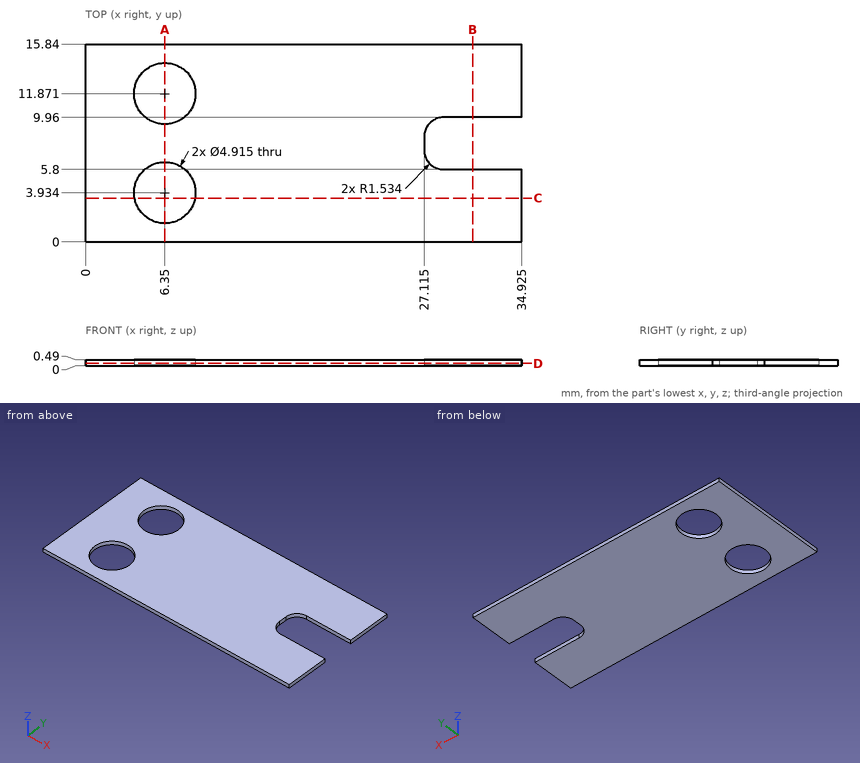
Check sheet for the drawn part. Datum: minimum x, y, z corner. Units: mm. Coordinates: 2 decimals unless noted, no trailing zeros. Loops run counter-clockwise (first coordinate to the right, second up) from the corner with the lowest first, then second, coordinate; pieces in that order, holes last. Notation, with made-up numbers: (-12, 49.5) -> (1, 49.5) arc R12 ccw to (1, 60.5) -> close; hole circle Ø5 at (-40, 45.25). An arc over 180 degrees is marked (long way). Answer as a JSON object with one key per item and string values. Group by question number.
Item 1: Depth check by flat-ended pin: pin 1 (4.5 mm diameter, centred on x = 6.35, y = 11.87, fed in from +Z). Enter the tip coordinate at first touch or a pass-through.
Item 2: Sectioned sample at B-B on x = 31. Record the boundary of the cut face in (y, z).
Item 3: Scan lines: probe 1 along Y at (x, z) = (6.35, 0.2); probe 2 along X at (y, z) = (4, 0.2) (1 decimal); probe 3 along X at (y, z) = (8.5, 0.3). Record each from-to range of solid material in increasing order.
Item 4: Sectioned sample at C-C on y = 3.5. Record the boundary of the cut face in (x, z) (1 decimal).
Item 5: Sectioned sample at A-A on x = 6.35. Record the boundary of the cut face in (y, z).
Item 6: Sectioned sample at D-D on z = 0.2. State how many separate pieces and enclosed holes the cut face has, plus the area to 3 significant figures.
Evaluation:
{
 "1": {"pin 1": "passes through"},
 "2": {"outline": "(0, 0) -> (5.8, 0) -> (5.8, 0.49) -> (0, 0.49) -> close; (9.96, 0) -> (15.84, 0) -> (15.84, 0.49) -> (9.96, 0.49) -> close"},
 "3": {"probe 1": "y = 0 to 1.48, 6.39 to 9.41, 14.33 to 15.84", "probe 2": "x = 0 to 3.9, 8.8 to 34.9", "probe 3": "x = 0 to 27.12"},
 "4": {"outline": "(0, 0) -> (3.9, 0) -> (3.9, 0.5) -> (0, 0.5) -> close; (8.8, 0) -> (34.9, 0) -> (34.9, 0.5) -> (8.8, 0.5) -> close"},
 "5": {"outline": "(0, 0) -> (1.48, 0) -> (1.48, 0.49) -> (0, 0.49) -> close; (6.39, 0) -> (9.41, 0) -> (9.41, 0.49) -> (6.39, 0.49) -> close; (14.33, 0) -> (15.84, 0) -> (15.84, 0.49) -> (14.33, 0.49) -> close"},
 "6": {"separate pieces": "1", "enclosed holes": "2", "area": "484 mm²"}
}
